Source: CAD feature listing. Evaluate the final solid. Frame: model axes, mm. A direction names the side the tool comes from. Give positions to 0.01 mm unless a question says otherwise; leave off trailing zeros. Order: outer loops, then holes, each group sorted by start corner. A loop starts at its lowest first (then second) coordinate and runs counter-clockwise, first axis right, second up.
1) Draft query along X for faces 1 (the face through (11.25, 0, -2)), 2 (the face through (0, -6, 8)), 3 (the face through (12.837, -0.059, 1.232)). Return one class per face: released by +X, released by -X, zero draft, split by the parting line, or undercut.
2) Section C-C, the plane x = 10. Return loops of the section in (y, z).
3) Material intervals for line 1 (Z direction, x = -2.5, y = -3.75); line 2 (X direction, y = 0, z = 0.8); line 3 (Z direction, x = -12.5, y = 0), sorted ascending.
4) Access query for faces 4 (the face through (2.39, 0.9, -13.24)), 5 (the face through (-0.5, 2.75, -6.7)), 6 (the face through (-0.5, -2.75, -6.7)), 7 (the face through (10, -5, -4.5)). Directions: +Z, -Z, +X, -X, +Y, -Y. A direction counts if a zero-diameter tool reaches every point of the face in a straight line with its end or side. Return the directions, or none.
5) Section D-D, the plane z = -2. Return loops of the section in (x, y).
6) Section A-A, the plane x = 13.5. Return loops of the section in (y, z).
7) First-contact query: P1, Ø0.7, axis at x = -0.5, z = -6, coming from the +Y side; P2, Ø2, axis at y = -1, z = -3, coming from the +X side; P3, Ø1.5, axis at x = -13, y = 3, coming from the +Z side. Flat tips, straight axial feed; report the tip coordinate or a pass-through.
8) Section B-B, the plane y = -2.25. Return loops of the section in (x, z), plus the area to 3 significant figures.
```python
from build123d import *

# Parameters (mm, degrees)
BOSS_EXTRUDE1_DEPTH = 2.5
SKETCH3_W           = 22.5
SKETCH3_H           = 12
BOSS_EXTRUDE2_DEPTH = 17.5
SKETCH4_W           = 22.5
SKETCH4_H           = 12
BOSS_EXTRUDE3_DEPTH = 4.5
BOSS_EXTRUDE4_DEPTH = 4.5
SKETCH6_R           = 3.5
BOSS_EXTRUDE5_DEPTH = 5
CUT_EXTRUDE1_START  = -1.5
SKETCH7_R           = 3.5
SKETCH7_R_2         = 3
CUT_EXTRUDE1_DEPTH  = 1.5


with BuildPart() as part:
    # Sketch2 → Boss-Extrude1 (new body)
    with BuildSketch(Plane.XY):
        with BuildLine():
            Line((-16.25, -6), (0, -6))
            Line((0, -6), (16.25, -6))
            Line((16.25, -6), (16.25, -0.5))
            Line((16.25, -0.5), (15.75, -0.5))
            ThreePointArc((15.75, -0.5), (12.835786438, 0), (15.75, 0.5))
            Line((15.75, 0.5), (16.25, 0.5))
            Line((16.25, 0.5), (16.25, 6))
            Line((16.25, 6), (0, 6))
            Line((0, 6), (-16.25, 6))
            Line((-16.25, 6), (-16.25, 0.5))
            Line((-16.25, 0.5), (-15.75, 0.5))
            ThreePointArc((-15.75, 0.5), (-12.835786438, 0), (-15.75, -0.5))
            Line((-15.75, -0.5), (-16.25, -0.5))
            Line((-16.25, -0.5), (-16.25, -6))
        make_face()
    extrude(amount=BOSS_EXTRUDE1_DEPTH)

    # Sketch3 → Boss-Extrude2 (add)
    with BuildSketch(Plane.XY.offset(2.5)):
        Rectangle(SKETCH3_W, SKETCH3_H)
    extrude(amount=BOSS_EXTRUDE2_DEPTH)

    # Sketch4 → Boss-Extrude3 (add)
    with BuildSketch(Plane(origin=(0, 0, 0), x_dir=(-1, 0, 0), z_dir=(0, 0, -1))):
        Rectangle(SKETCH4_W, SKETCH4_H)
    extrude(amount=BOSS_EXTRUDE3_DEPTH)

    # Sketch5 → Boss-Extrude4 (add)
    with BuildSketch(Plane(origin=(0, 0, -4.5), x_dir=(-1, 0, 0), z_dir=(0, 0, -1))):
        with BuildLine():
            Line((1, 2.75), (0.082682252, 2.75))
            ThreePointArc((0.082682252, 2.75), (-11.25, 0), (0.082682252, -2.75))
            Line((0.082682252, -2.75), (1, -2.75))
            ThreePointArc((1, -2.75), (3.75, 0), (1, 2.75))
        make_face()
    extrude(amount=BOSS_EXTRUDE4_DEPTH)

    # Sketch6 → Boss-Extrude5 (add)
    with BuildSketch(Plane(origin=(0, 0, -9), x_dir=(-1, 0, 0), z_dir=(0, 0, -1))):
        with Locations((-5.25, 0)):
            Circle(SKETCH6_R)
    extrude(amount=BOSS_EXTRUDE5_DEPTH)

    # Sketch7 → Cut-Extrude1 (cut)
    with BuildSketch(Plane(origin=(0, 0, -14), x_dir=(-1, 0, 0), z_dir=(0, 0, -1)).offset(CUT_EXTRUDE1_START)):
        with Locations((-5.25, 0)):
            Circle(SKETCH7_R)
        with Locations((-5.25, 0)):
            Circle(SKETCH7_R_2, mode=Mode.SUBTRACT)
    extrude(amount=CUT_EXTRUDE1_DEPTH, mode=Mode.SUBTRACT)


solid = part.part
```
From the geometry:
1. face 1: released by +X
1. face 2: zero draft
1. face 3: undercut
2. outline: (-6, -4.5) - (-3.67, -4.5) - (-3.67, -9) - (3.67, -9) - (3.67, -4.5) - (6, -4.5) - (6, 20) - (-6, 20) - close
3. line 1: z = -4.5 to 20
3. line 2: x = -12.84 to 12.84
3. line 3: z = 0 to 2.5
4. face 4: -Z
4. face 5: -Z, -X, +Y
4. face 6: -Z, -X, -Y
4. face 7: -Z, +X, -Y
5. outline: (-11.25, -6) - (11.25, -6) - (11.25, 6) - (-11.25, 6) - close
6. outline: (-6, 0) - (-1.25, 0) - (-1.25, 2.5) - (-6, 2.5) - close; (1.25, 0) - (6, 0) - (6, 2.5) - (1.25, 2.5) - close
7. P1: stops at y = 2.75
7. P2: stops at x = 11.25
7. P3: stops at z = 2.5
8. outline: (-16.25, 0) - (-11.25, 0) - (-11.25, -4.5) - (-2.58, -4.5) - (-2.58, -9) - (2.57, -9) - (2.57, -12.5) - (3.27, -12.5) - (3.27, -14) - (7.23, -14) - (7.23, -12.5) - (7.93, -12.5) - (7.93, -9) - (10.81, -9) - (10.81, -4.5) - (11.25, -4.5) - (11.25, 0) - (16.25, 0) - (16.25, 2.5) - (11.25, 2.5) - (11.25, 20) - (-11.25, 20) - (-11.25, 2.5) - (-16.25, 2.5) - close
8. area: 661 mm2
